```python
from build123d import *

# Parameters (mm, degrees)
F0_W     = 869.95
F0_H     = 406.4
F1_DEPTH = 88.9
F2_SIZE  = 63.5
F3_T     = -2.6416
F5_D     = 9.525
F6_D     = 12.7
F7_D     = 15.875
F8_D     = 19.05
F9_D     = 22.225
F10_D    = 25.4
F11_D    = 28.575
F12_D    = 31.75


with BuildPart() as f1:
    # F0 (on Top) → F1 (new body)
    with BuildSketch(Plane.XY):
        with Locations((434.975, -203.2)):
            Rectangle(F0_W, F0_H)
    extrude(amount=F1_DEPTH)

    # F2
    f2_edges = [f1.edges().sort_by_distance(p)[0] for p in [
        (0, -203.2, 0),
    ]]
    chamfer(f2_edges, length=F2_SIZE)

    # F3
    f3_openings = [f1.faces().sort_by_distance(p)[0] for p in [
        (434.975, -203.2, 88.9),
        (446.05124, -406.4, 45.073216),
        (446.05124, 0, 45.073216),
        (869.95, -203.2, 44.45),
    ]]
    offset(amount=F3_T, openings=f3_openings)

    # F5 (through all)
    with Locations(Plane.XY.offset(2.6416)):
        with Locations((97.79, -50.8), (97.79, -127), (97.79, -203.2), (97.79, -279.4), (97.79, -355.6)):
            Hole(F5_D / 2)

    # F6 (through all)
    with Locations(Plane.XY.offset(2.6416)):
        with Locations((194.31, -50.8), (194.31, -127), (194.31, -203.2), (194.31, -279.4), (194.31, -355.6)):
            Hole(F6_D / 2)

    # F7 (through all)
    with Locations(Plane.XY.offset(2.6416)):
        with Locations((290.83, -50.8), (290.83, -127), (290.83, -203.2), (290.83, -279.4), (290.83, -355.6)):
            Hole(F7_D / 2)

    # F8 (through all)
    with Locations(Plane.XY.offset(2.6416)):
        with Locations((387.35, -355.6), (387.35, -279.4), (387.35, -203.2), (387.35, -127), (387.35, -50.8)):
            Hole(F8_D / 2)

    # F9 (through all)
    with Locations(Plane.XY.offset(2.6416)):
        with Locations((483.87, -355.6), (483.87, -279.4), (483.87, -203.2), (483.87, -127), (483.87, -50.8)):
            Hole(F9_D / 2)

    # F10 (through all)
    with Locations(Plane.XY.offset(2.6416)):
        with Locations((580.39, -355.6), (580.39, -279.4), (580.39, -203.2), (580.39, -127), (580.39, -50.8)):
            Hole(F10_D / 2)

    # F11 (through all)
    with Locations(Plane.XY.offset(2.6416)):
        with Locations((676.91, -355.6), (676.91, -279.4), (676.91, -203.2), (676.91, -127), (676.91, -50.8)):
            Hole(F11_D / 2)

    # F12 (through all)
    with Locations(Plane.XY.offset(2.6416)):
        with Locations((773.43, -355.6), (773.43, -279.4), (773.43, -203.2), (773.43, -127), (773.43, -50.8)):
            Hole(F12_D / 2)


solid = f1.part
```
Read the model definition and answer for the solid it produces. Units are mm, in the model's axes. Give positions to 0.01 mm unless a question says otherwise; leave off trailing zeros. Write each loop counter-clockwise with the first axis right and the second up, starting at its lowest first coordinate (ties: lowest second). Pieces come first, ordered by that corner, then holes. Notation, with made-up numbers: (78, 53.5) -> (136, 53.5) arc R14 cw to (136, 75.5) -> close; hole circle Ø4 at (-23, 37.25). An arc over 180 degrees is marked (long way). Answer in a Markdown table with one row per item.
1) Section A-A on x = 483.87 is taken. Give the vertices of the cut face in (y, z), plus the area to 3 significant figures.
Results list:
| item | result |
|---|---|
| outline | (-406.4, 0) -> (-366.71, 0) -> (-366.71, 2.64) -> (-406.4, 2.64) -> close; (-344.49, 0) -> (-290.51, 0) -> (-290.51, 2.64) -> (-344.49, 2.64) -> close; (-268.29, 0) -> (-214.31, 0) -> (-214.31, 2.64) -> (-268.29, 2.64) -> close; (-192.09, 0) -> (-138.11, 0) -> (-138.11, 2.64) -> (-192.09, 2.64) -> close; (-115.89, 0) -> (-61.91, 0) -> (-61.91, 2.64) -> (-115.89, 2.64) -> close; (-39.69, 0) -> (0, 0) -> (0, 2.64) -> (-39.69, 2.64) -> close |
| area | 780 mm^2 |
2) Section B-B on y = -240 is taken. Give the vertices of the cut face in (x, z), plus the area to 3 significant figures.
Results list:
| item | result |
|---|---|
| outline | (0, 63.5) -> (63.5, 0) -> (869.95, 0) -> (869.95, 2.64) -> (64.59, 2.64) -> (2.64, 64.59) -> (2.64, 88.9) -> (0, 88.9) -> close |
| area | 2,430 mm^2 |
3) Straight lines are drawn through the part: line 1 (Y direction, x = 290, z = 1); line 2 (Y direction, x = 387.35, z = 1.45) (3 decimals); line 3 (Z direction, x = 553.5, y = -208.5). For each, find the intervals that lie inside material, in ascending order. Write a range as [from, to].
Results list:
| item | result |
|---|---|
| line 1 | [-406.4, -363.49], [-347.71, -287.29], [-271.51, -211.09], [-195.31, -134.89], [-119.11, -58.69], [-42.91, 0] |
| line 2 | [-406.4, -365.125], [-346.075, -288.925], [-269.875, -212.725], [-193.675, -136.525], [-117.475, -60.325], [-41.275, 0] |
| line 3 | [0, 2.64] |
4) Each of these flat-tipped pins is pushed along its axis until it touches: pin 1 Ø16.5 at (x, y) = (194.31, -127) entering from +Z; pin 2 Ø15 at (x, y) = (580.39, -127) entering from -Z; pin 3 Ø1 at (y, z) = (-291.5, 52) entering from +X; pin 4 Ø2 at (y, z) = (-253, 29.5) entering from +X. Where does it stop, or does it pass through?
Results list:
| item | result |
|---|---|
| pin 1 | z = 2.64 |
| pin 2 | through |
| pin 3 | x = 15.74 |
| pin 4 | x = 38.74 |
5) Section D-D on x = 77 is taken. Give the vertices of the cut face in (y, z).
Results list:
| item | result |
|---|---|
| outline | (-406.4, 0) -> (0, 0) -> (0, 2.64) -> (-406.4, 2.64) -> close |
6) Section C-C on x = 290.83 is taken. Give the vertices of the cut face in (y, z).
Results list:
| item | result |
|---|---|
| outline | (-406.4, 0) -> (-363.54, 0) -> (-363.54, 2.64) -> (-406.4, 2.64) -> close; (-347.66, 0) -> (-287.34, 0) -> (-287.34, 2.64) -> (-347.66, 2.64) -> close; (-271.46, 0) -> (-211.14, 0) -> (-211.14, 2.64) -> (-271.46, 2.64) -> close; (-195.26, 0) -> (-134.94, 0) -> (-134.94, 2.64) -> (-195.26, 2.64) -> close; (-119.06, 0) -> (-58.74, 0) -> (-58.74, 2.64) -> (-119.06, 2.64) -> close; (-42.86, 0) -> (0, 0) -> (0, 2.64) -> (-42.86, 2.64) -> close |
7) Determine the mould class of faces 1 (the flat face through (433, 0, 1)), 2 (the flat face through (0, -206, 76)), 3 (the cylindrical face through (758.766, -209.28, 1.302)), 4 (the cylindrical face through (382.95, -211.65, 1.3)) for opening direction X: released by +X, released by -X, zero draft, split by the parting line, or undercut.
Results list:
| item | result |
|---|---|
| face 1 | zero draft |
| face 2 | released by -X |
| face 3 | undercut |
| face 4 | undercut |
